The model under review builds one solid part; all positions refer to its coordinate system, in mm. A direction names the side the tool comes from. Coordinates: 2 decimals unless noted, no trailing zeros. Order: outer loops, then holes, each group sorted by start corner. A loop starts at its lowest first (then second) coordinate and runs counter-clockwise, first axis right, second up. Notation, with made-up numbers: (13.25, -3.5) - (47.25, -3.5) arc R15 cw to (47.25, 5.5) - close; hole circle Ø4 at (39, -14). An arc over 180 degrees is marked (long way). Answer in a Markdown table with one row per item.
```python
from build123d import *

# Parameters (mm, degrees)
SKETCH2_W           = 914.4
SKETCH2_H           = 457.2
BOSS_EXTRUDE2_DEPTH = 12.7
SKETCH1_W           = 914.4
SKETCH1_H           = 457.2
SKETCH1_W_2         = 876.3
SKETCH1_H_2         = 419.1
BOSS_EXTRUDE3_DEPTH = 88.9


with BuildPart() as part:
    # Sketch2 → Boss-Extrude2 (new body)
    with BuildSketch(Plane(origin=(0, 0, 0), x_dir=(1, 0, 0), z_dir=(0, 1, 0))):
        with Locations((457.2, 228.6)):
            Rectangle(SKETCH2_W, SKETCH2_H)
    extrude(amount=-BOSS_EXTRUDE2_DEPTH)

    # Sketch1 → Boss-Extrude3 (add)
    with BuildSketch(Plane(origin=(0, 0, 0), x_dir=(1, 0, 0), z_dir=(0, 1, 0))):
        with Locations((457.2, 228.6)):
            Rectangle(SKETCH1_W, SKETCH1_H)
        with Locations((457.2, 228.6)):
            Rectangle(SKETCH1_W_2, SKETCH1_H_2, mode=Mode.SUBTRACT)
    extrude(amount=BOSS_EXTRUDE3_DEPTH)


solid = part.part
```
Item 1: We need section B-B, the plane z = -239.5. Write out the cut boundary in (x, y).
Check values:
| item | result |
|---|---|
| outline | (0, -12.7) - (914.4, -12.7) - (914.4, 88.9) - (895.35, 88.9) - (895.35, 0) - (19.05, 0) - (19.05, 88.9) - (0, 88.9) - close |
Item 2: Tool access review of faces 4 (the face through (895.35, 44, -226)), 5 (the face through (320, 88.9, -450)): name each direction out of +Z, -Z, +X, -X, +Y, -Y from which nothing blocks a thin tool from reaching the whole face with its end or side.
Check values:
| item | result |
|---|---|
| face 4 | +Y |
| face 5 | +Z, -Z, +X, -X, +Y |
Item 3: We need section A-A, the plane y = 25.5. Write out the cut boundary in (x, z).
Check values:
| item | result |
|---|---|
| outline | (0, -457.2) - (914.4, -457.2) - (914.4, 0) - (0, 0) - close; hole (19.05, -438.15) - (895.35, -438.15) - (895.35, -19.05) - (19.05, -19.05) - close |
Item 4: Mouldability with a two-part tool opening along X and no side actions: class faces 1 (the face through (0, 37, -225)), 2 (the face through (451, 37, -457.2)), 3 (the face through (451, 0, -232)) as +X half, -X half, draft (parallel to the pull), parting line (faces both ways), or undercut.
Check values:
| item | result |
|---|---|
| face 1 | -X half |
| face 2 | draft |
| face 3 | undercut |
Item 5: Clearance check with a flat-ended pin moving along its axis: pin 1 Ø10 at (x, z) = (380, -173.5) entering from +Y. State where the tip first meets the part, or that it passes through.
Check values:
| item | result |
|---|---|
| pin 1 | y = 0 |
Item 6: We need section C-C, the plane x = 104. Write out the cut boundary in (y, z), then the cut area to 3 significant figures.
Check values:
| item | result |
|---|---|
| outline | (-12.7, -457.2) - (88.9, -457.2) - (88.9, -438.15) - (0, -438.15) - (0, -19.05) - (88.9, -19.05) - (88.9, 0) - (-12.7, 0) - close |
| area | 9,190 mm^2 |
Item 7: To check wall thickness, follow line 1 (X direction, y = 3, z = -105); line 2 (Z direction, x = 548, y = 47.5); line 3 (Y direction, x = 306.5, z = -193.5). State the ranges of each line that lie inside material, in increasing order. Write a range as from..to.
Check values:
| item | result |
|---|---|
| line 1 | 0..19.05, 895.35..914.4 |
| line 2 | -457.2..-438.15, -19.05..0 |
| line 3 | -12.7..0 |
